from build123d import *

# Parameters (mm, degrees)
SKETCH1_R               = 127
SKETCH1_R_2             = 117.475
BOSS_EXTRUDE1_DEPTH     = 50.8
SKETCH1_3_R             = 130.175
SKETCH1_3_R_2           = 127
BOSS_EXTRUDE2_DEPTH     = 254
SKETCH1_4_R             = 139.7
SKETCH1_4_R_2           = 130.175
BOSS_EXTRUDE3_DEPTH     = 6.35
SKETCH2_W               = 130.175
SKETCH2_H               = 127
CUT_EXTRUDE1_DEPTH      = 235.864173513
CUT_EXTRUDE1_DEPTH_BACK = 235.864173513


with BuildPart() as part:
    # Sketch1 → Boss-Extrude1 (new body)
    with BuildSketch(Plane(origin=(0, 0, 0), x_dir=(1, 0, 0), z_dir=(0, 1, 0))):
        with Locations(Location((0, 0, 0), (0, 0, 270))):
            Circle(SKETCH1_R)
        with Locations(Location((0, 0, 0), (0, 0, 270))):
            Circle(SKETCH1_R_2, mode=Mode.SUBTRACT)
    extrude(amount=BOSS_EXTRUDE1_DEPTH)

    # Sketch1_3 → Boss-Extrude2 (add)
    with BuildSketch(Plane(origin=(0, 0, 0), x_dir=(1, 0, 0), z_dir=(0, 1, 0))):
        with Locations(Location((0, 0, 0), (0, 0, 270))):
            Circle(SKETCH1_3_R)
        with Locations(Location((0, 0, 0), (0, 0, 270))):
            Circle(SKETCH1_3_R_2, mode=Mode.SUBTRACT)
    extrude(amount=BOSS_EXTRUDE2_DEPTH)

    # Sketch1_4 → Boss-Extrude3 (add)
    with BuildSketch(Plane(origin=(0, 0, 0), x_dir=(1, 0, 0), z_dir=(0, 1, 0))):
        with Locations(Location((0, 0, 0), (0, 0, 270))):
            Circle(SKETCH1_4_R)
        with Locations(Location((0, 0, 0), (0, 0, 270))):
            Circle(SKETCH1_4_R_2, mode=Mode.SUBTRACT)
    extrude(amount=BOSS_EXTRUDE3_DEPTH)

    # Sketch2 → Cut-Revolve4 (revolve, cut)
    with BuildSketch(Plane(origin=(0, 0, 0), x_dir=(0, 0, -1), z_dir=(1, 0, 0)), mode=Mode.PRIVATE) as cut_revolve4_sk:
        with Locations((-65.0875, 190.5)):
            Rectangle(SKETCH2_W, SKETCH2_H)
    revolve(cut_revolve4_sk.sketch.rotate(Axis((0, 254, 0), (0, -1, 0)), 180), axis=Axis((0, 254, 0), (0, -1, 0)), mode=Mode.SUBTRACT)

    # Sketch3 → Cut-Extrude1 (cut, two sides: drawn at the far end of the back side and taken through both)
    with BuildSketch(Plane(origin=(0, 0, 0), x_dir=(0, 0, -1), z_dir=(1, 0, 0)).offset(-CUT_EXTRUDE1_DEPTH_BACK)):
        Polygon((-76.2, 127), (76.2, 127), (0, 50.8), align=None)
    extrude(amount=CUT_EXTRUDE1_DEPTH + CUT_EXTRUDE1_DEPTH_BACK, mode=Mode.SUBTRACT)


solid = part.part
Verification items for the finished model (mm, model axes). A direction names the side the tool comes from. Coordinates: 2 decimals unless noted, no trailing zeros. Loops run counter-clockwise (first coordinate to the right, second up) from the corner with the lowest first, then second, coordinate; pieces in that order, holes last. Notation, with made-up numbers: (85.5, 38.5) -> (109.5, 38.5) arc R24 cw to (109.5, 74.5) -> close; hole circle Ø2 at (-9, -14). An arc over 180 degrees is marked (long way). Answer as a JSON object with one key per item and string values. Group by question number.
Item 1: Depth check by flat-ended pin: pin 1 (4 mm diameter, centred on x = -95, y = 37.5, fed in from +Z); pin 2 (1 mm diameter, centred on x = 85, y = 25, fed in from -Z); pin 3 (5 mm diameter, centred on y = 90.5, z = 110.5, fed in from +X). Enter the tip coordinate at first touch or a pass-through.
Item 2: Sectioned sample at A-A on x = 0. Record the boundary of the cut face in (y, z) (3 decimals), plus the area to 3 significant figures.
Item 3: Sectioned sample at C-C on z = -88. Record the boundary of the cut face in (x, y).
Item 4: Scan lines: probe 1 along Z at (x, y) = (-1, 23); probe 2 along X at (y, z) = (40, 0) (3 decimals); probe 3 along X at (y, z) = (63, 48.5). Record each from-to range of solid material in increasing order.
Item 5: Mould release check, pull along X, two halves, no side actions. Record for faces 1 (the cylindrical face through (2.79, 88.37, -126.97)), 2 (the cylindrical face through (109.764, 65.83, 69.981)), 3 (the flat face through (62.7, 6.35, -114.5)), 4 (the flat face through (-37, 50.8, 112)): +X half, -X half, draft (parallel to the pull), parting line (faces both ways), or undercut.
Item 6: Sectioned sample at D-D on y = 34. Record the boundary of the cut face in (x, z) (3 decimals), plus the area to 3 significant figures.
Item 7: Sectioned sample at B-B on y = 64.5. Record the boundary of the cut face in (x, z) (3 decimals), plus the area to 3 significant figures.
Item 8: Tool access check on faces 5 (the flat face through (121.1, 91.5, 40.7)), 6 (the cylindrical face through (-136.38, 3.13, -30.28)), 7 (the cylindrical face through (-2.79, 88.37, 126.97)). Record the directions out of +Z, -Z, +X, -X, +Y, -Y that give a thin tool (end or side, any length) a straight path to the whole face; none if there is none.
Evaluation:
{
 "1": {"pin 1": "stops at z = 91.09", "pin 2": "stops at z = -99.02", "pin 3": "stops at x = 72.67"},
 "2": {"outline": "(0, -139.7) -> (6.35, -139.7) -> (6.35, -130.175) -> (127, -130.175) -> (127, -127) -> (50.8, -127) -> (50.8, -117.475) -> (0, -117.475) -> close; (0, 117.475) -> (50.8, 117.475) -> (50.8, 127) -> (127, 127) -> (127, 130.175) -> (6.35, 130.175) -> (6.35, 139.7) -> (0, 139.7) -> close", "area": "1,900 mm²"},
 "3": {"outline": "(-108.5, 0) -> (-77.82, 0) -> (-77.82, 50.8) -> (-91.57, 50.8) -> (-91.57, 127) -> (-95.92, 127) -> (-95.92, 6.35) -> (-108.5, 6.35) -> close; (77.82, 0) -> (108.5, 0) -> (108.5, 6.35) -> (95.92, 6.35) -> (95.92, 127) -> (91.57, 127) -> (91.57, 50.8) -> (77.82, 50.8) -> close"},
 "4": {"probe 1": "z = -130.17 to -117.47, 117.47 to 130.17", "probe 2": "x = -130.175 to -117.475, 117.475 to 130.175", "probe 3": "x = -120.8 to -117.37, 117.37 to 120.8"},
 "5": {"face 1": "undercut", "face 2": "parting line", "face 3": "draft", "face 4": "undercut"},
 "6": {"outline": "circle Ø260.35 at (0, 0); hole circle Ø234.95 at (0, 0)", "area": "9,880 mm²"},
 "7": {"outline": "(-129.452, -13.7) arc R130.175 ccw to (129.452, -13.7) -> (126.259, -13.7) arc R127 cw to (-126.259, -13.7) -> close; (-129.452, 13.7) -> (-126.259, 13.7) arc R127 cw to (126.259, 13.7) -> (129.452, 13.7) arc R130.175 ccw to start", "area": "2,390 mm²"},
 "8": {"face 5": "+X, -X, +Y", "face 6": "+Y, -Y", "face 7": "+Y"}
}
